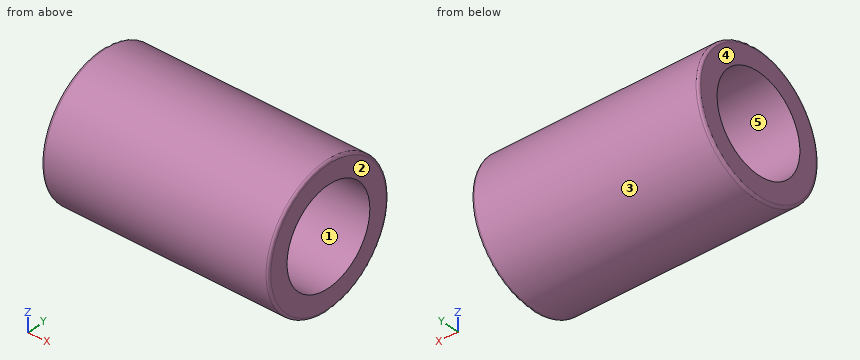
Autodesk Inventor part; units mm, degrees
ref_plane "YZ Plane" through (0, 0, 0) normal (1, 0, 0) x (0, 1, 0)
ref_plane "XZ Plane" through (0, 0, 0) normal (0, 1, 0) x (-1, 0, 0)
ref_plane "XY Plane" through (0, 0, 0) normal (0, 0, 1) x (1, 0, 0)
sketch "Sketch1" plane through (0, 0, 0) normal (0, 1, 0) x (-1, 0, 0)
  point P0 (0, 0)
sketch "Sketch2" plane through (0, 0, 0) normal (0, 1, 0) x (-1, 0, 0)
  line L0 (29.6036, 0) -> (-33.9054, 0)
  circle A0 centre (0, -19) radius 1.5
  point P0 (0, 0)
  dimension "d0" = 19
  dimension "d1" = 3
revolve "Revolution1" add sketch "Sketch2" angle 360 about axis through (-29.6036, 0, 0) along (1, 0, 0)
sketch "Sketch3" plane through (0, 0, 0) normal (1, 0, 0) x (0, 1, 0)
  circle A0 centre (0, 0) radius 19
  circle A1 centre (0, 0) radius 27.5
  dimension "d3" = 38
  dimension "d4" = 55
extrude "Extrusion1" add sketch "Sketch3" along normal mid plane 90
fillet "Fillet1" radius 1 1 edges at (45, -27.5, 0)
fillet "Fillet2" radius 1 1 edges at (-45, -27.5, 0)
properties part number "linker"
Can you work these out from the model? Positions are in its coordinate system, mm. Face numbers are marked on the shaded views. A direction names the side the tool comes from. Round coordinates to 2 decimals unless told otherwise and drop trailing zeros. Loops run counter-clockwise (first coordinate to the right, second up) from the corner with the lowest first, then second, coordinate; pieces in that order, holes last. Notation, with made-up numbers: (22, -29) - (59, -29) arc R15 ccw to (59, -17) - close; hole circle Ø11 at (-1.5, 30.25). An arc over 180 degrees is marked (long way). Use CSV: the item, a comma, the result in double quotes. Start each with the question number.
1) If we section it at C-C on x = 38: Write out the boundary of the cut face in (y, z), plus the area to 3 significant figures.
2) We'd pull the mould along Z, two halves only. Please class the marked faces 3, 4 and 5: released by +Z, released by -Z, zero draft, split by the parting line, or undercut.
3) Please list where these lines run through material, in increasing order: probe 1 along Z at (x, y) = (-14, 0); probe 2 along Z at (x, y) = (-18, -15); probe 3 along Y at (x, z) = (25, 14.5). Write a range as [from, to].
4) If we section it at A-A on y = 0: Write out the boundary of the cut face in (x, z).
5) For the marked faces 1 and 2, which set-ups out of +Z, -Z, +X, -X, +Y, -Y let a thin tool reach every point of the face, with its end or its side?
6) For pin 1 Ø1.5 at (x, z) = (-14.5, 17.5) entering from +Y; pin 2 Ø3 at (x, y) = (-33, -12.5) entering from +Z; pin 3 Ø1.5 at (x, y) = (7.5, -4.5) entering from +Z, each with a flat end and sliding along its axis, tell me the tip position at first contact or that it passes through.
Geometry results:
1,outline,"circle Ø55 at (0, 0); hole circle Ø38 at (0, 0)"
1,area,"1,240 mm2"
2,face 3,"split by the parting line"
2,face 4,"zero draft"
2,face 5,"undercut"
3,probe 1,"z = [-27.5, -19], [19, 27.5]"
3,probe 2,"z = [-23.05, -11.66], [11.66, 23.05]"
3,probe 3,"y = [-23.37, -12.28], [12.28, 23.37]"
4,outline,"(-45, -26.5) arc R1 ccw to (-44, -27.5) - (44, -27.5) arc R1 ccw to (45, -26.5) - (45, -19) - (1.5, -19) arc R1.5 ccw to (-1.5, -19) - (-45, -19) - close; (-45, 19) - (-1.5, 19) arc R1.5 ccw to (1.5, 19) - (45, 19) - (45, 26.5) arc R1 ccw to (44, 27.5) - (-44, 27.5) arc R1 ccw to (-45, 26.5) - close"
5,face 1,"+X"
5,face 2,"+Z, -Z, +X, +Y, -Y"
6,pin 1,"stops at y = 21.81"
6,pin 2,"stops at z = 25.2"
6,pin 3,"stops at z = 27.24"
